The model under review builds one solid part; all positions refer to its coordinate system, in mm. A direction names the side the tool comes from. Give positions to 0.01 mm unless a question says otherwise; leave off trailing zeros. Write each loop counter-clockwise with the first axis right and the second up, starting at its lowest first coordinate (ties: lowest second). Pieces come first, ordered by that corner, then holes.
from build123d import *

# Parameters (mm, degrees)
SKETCH3_R             = 25.4
SKETCH3_R_2           = 20.32
BOSS_EXTRUDE1_DEPTH   = 25.4
BOSS_EXTRUDE3_START   = 7
SKETCH4_R             = 5
BOSS_EXTRUDE3_DEPTH   = 5
BOSS_EXTRUDE3_2_DEPTH = 5
BOSS_EXTRUDE4_START   = -7
SKETCH4_2_R           = 5
BOSS_EXTRUDE4_DEPTH   = 5
BOSS_EXTRUDE4_2_DEPTH = 5
BOSS_EXTRUDE5_DEPTH   = 25.4


with BuildPart() as part:
    # Sketch3 → Boss-Extrude1 (new, symmetric)
    with BuildSketch(Plane(origin=(0, 0, 0), x_dir=(0, 0, -1), z_dir=(1, 0, 0))):
        Circle(SKETCH3_R)
        Circle(SKETCH3_R_2, mode=Mode.SUBTRACT)
    extrude(amount=BOSS_EXTRUDE1_DEPTH, both=True)



with BuildPart() as body_2:
    # Sketch4 → Boss-Extrude3 (new body)
    with BuildSketch(Plane.XY.offset(BOSS_EXTRUDE3_START)):
        with BuildLine():
            Line((-25.4, 25.4), (-9.806723533, 103.556571886))
            ThreePointArc((-9.806723533, 103.556571886), (0, 111.6), (9.806723533, 103.556571886))
            Line((9.806723533, 103.556571886), (25.4, 25.4))
            Line((25.4, 25.4), (-25.4, 25.4))
        make_face()
        with Locations((0, 101.6)):
            Circle(SKETCH4_R, mode=Mode.SUBTRACT)
    extrude(amount=BOSS_EXTRUDE3_DEPTH)


with BuildPart() as body_3:
    # Sketch4 → Boss-Extrude3 2 (new body)
    with BuildSketch(Plane.XY.offset(BOSS_EXTRUDE3_START)):
        with BuildLine():
            Line((-25.4, -25.4), (-9.806723533, -103.556571886))
            ThreePointArc((-9.806723533, -103.556571886), (0, -111.6), (9.806723533, -103.556571886))
            Line((9.806723533, -103.556571886), (25.4, -25.4))
            Line((25.4, -25.4), (-25.4, -25.4))
        make_face()
        with Locations((0, -101.6)):
            Circle(SKETCH4_R, mode=Mode.SUBTRACT)
    extrude(amount=BOSS_EXTRUDE3_2_DEPTH)


with BuildPart() as body_4:
    # Sketch4<2> → Boss-Extrude4 (new body)
    with BuildSketch(Plane.XY.offset(BOSS_EXTRUDE4_START)):
        with BuildLine():
            Line((-25.4, 25.4), (-9.806723533, 103.556571886))
            ThreePointArc((-9.806723533, 103.556571886), (0, 111.6), (9.806723533, 103.556571886))
            Line((9.806723533, 103.556571886), (25.4, 25.4))
            Line((25.4, 25.4), (-25.4, 25.4))
        make_face()
        with Locations((0, 101.6)):
            Circle(SKETCH4_2_R, mode=Mode.SUBTRACT)
    extrude(amount=-BOSS_EXTRUDE4_DEPTH)


with BuildPart() as body_5:
    # Sketch4<2> → Boss-Extrude4 2 (new body)
    with BuildSketch(Plane.XY.offset(BOSS_EXTRUDE4_START)):
        with BuildLine():
            Line((-25.4, -25.4), (-9.806723533, -103.556571886))
            ThreePointArc((-9.806723533, -103.556571886), (0, -111.6), (9.806723533, -103.556571886))
            Line((9.806723533, -103.556571886), (25.4, -25.4))
            Line((25.4, -25.4), (-25.4, -25.4))
        make_face()
        with Locations((0, -101.6)):
            Circle(SKETCH4_2_R, mode=Mode.SUBTRACT)
    extrude(amount=-BOSS_EXTRUDE4_2_DEPTH)


with BuildPart() as part_1:
    add(part.part)

    add(body_2.part)  # Boss-Extrude5 merges body 2

    add(body_3.part)  # Boss-Extrude5 merges body 3

    add(body_4.part)  # Boss-Extrude5 merges body 4

    add(body_5.part)  # Boss-Extrude5 merges body 5
    # Sketch5 → Boss-Extrude5 (add, symmetric)
    with BuildSketch(Plane(origin=(0, 0, 0), x_dir=(0, 0, -1), z_dir=(1, 0, 0))):
        with BuildLine():
            Line((12, -25.4), (7, -25.4))
            Line((7, -25.4), (7, -24.416387939))
            ThreePointArc((7, -24.416387939), (9.554057075, -23.534655158), (12, -22.386603137))
            Line((12, -22.386603137), (12, -25.4))
        make_face()
        with BuildLine():
            Line((-12, -25.4), (-7, -25.4))
            Line((-7, -25.4), (-7, -24.416387939))
            ThreePointArc((-7, -24.416387939), (-9.554057075, -23.534655158), (-12, -22.386603137))
            Line((-12, -22.386603137), (-12, -25.4))
        make_face()
        with BuildLine():
            Line((12, 25.4), (7, 25.4))
            Line((7, 25.4), (7, 24.416387939))
            ThreePointArc((7, 24.416387939), (9.554057075, 23.534655158), (12, 22.386603137))
            Line((12, 22.386603137), (12, 25.4))
        make_face()
        with BuildLine():
            Line((-12, 25.4), (-7, 25.4))
            Line((-7, 25.4), (-7, 24.416387939))
            ThreePointArc((-7, 24.416387939), (-9.554057075, 23.534655158), (-12, 22.386603137))
            Line((-12, 22.386603137), (-12, 25.4))
        make_face()
    extrude(amount=BOSS_EXTRUDE5_DEPTH, both=True)


solid = part_1.part
1) Consider section C-C, the plane z = -2.5. Give the boundary of the cut face in (x, y).
2) Consider section B-B, the plane y = 31. Give the boundary of the cut face in (x, z), then the cut area to 3 significant figures.
3) The part is to be moulded in two halves that separate along Y. For faces 1 (the cylindrical face through (2.688, 105.816, 9.465)), 2 (the cylindrical face through (-0.2, -111.6, 9.5)), 3 (the flat face through (17.5, 65, -9.5)), say which applies: +Y half, -Y half, draft (parallel to the pull), parting line (faces both ways), or undercut.
4) Tool access review of faces 4 (the flat face through (0, -56, -12)), 5 (the cylindrical face through (-0.2, 111.6, -9.5)): name each direction out of +Z, -Z, +X, -X, +Y, -Y from which nothing blocks a thin tool from reaching the whole face with its end or side.
5) Consider section D-D, the plane z = 9. Give the boundary of the cut face in (x, y), then the cut area to 3 significant figures.
6) To check wall thickness, follow probe 1 along Z at (x, y) = (6, -57); probe 2 along Y at (x, z) = (-2.5, 11); probe 3 along Y at (x, z) = (11.5, 0). State the ranges of each line that lie inside material, in increasing order.
7) Insertion check: pin 1 (11.5 mm diameter, centred on x = 0, y = 101.6, fed in from +Z); pin 2 (12 mm diameter, centred on x = -12, y = 70, fed in from -Z); pin 3 (3 mm diameter, centred on y = 67.5, z = -8, fed in from -X). Each pin has a flat end and moves straight along its axis. Give the tip position at first contact, or say it passes through.
8) Consider section A-A, the plane x = 0. State how many separate pieces and enclosed holes the cut face has, then the cut area to 3 significant figures.
Answer block:
1. outline: (-25.4, -25.28) - (25.4, -25.28) - (25.4, -20.17) - (-25.4, -20.17) - close; (-25.4, 20.17) - (25.4, 20.17) - (25.4, 25.28) - (-25.4, 25.28) - close
2. outline: (-24.28, -12) - (24.28, -12) - (24.28, -7) - (-24.28, -7) - close; (-24.28, 7) - (24.28, 7) - (24.28, 12) - (-24.28, 12) - close
2. area: 486 mm2
3. face 1: undercut
3. face 2: -Y half
3. face 3: +Y half
4. face 4: -Z, +X, -X, -Y
4. face 5: +Z, -Z, +Y
5. outline: (-25.4, -25.4) - (-9.81, -103.56) arc R10 ccw to (9.81, -103.56) - (25.4, -25.4) - (25.4, -18.22) - (-25.4, -18.22) - close; (-25.4, 18.22) - (25.4, 18.22) - (25.4, 25.4) - (9.81, 103.56) arc R10 ccw to (-9.81, 103.56) - (-25.4, 25.4) - close; hole circle Ø10 at (0, -101.6); hole circle Ø10 at (0, 101.6)
5. area: 6,310 mm2
6. probe 1: z = -12 to -7, 7 to 12
6. probe 2: y = -111.28 to -105.93, -97.27 to -17.09, 17.09 to 97.27, 105.93 to 111.28
6. probe 3: y = -25.4 to -20.32, 20.32 to 25.4
7. pin 1: stops at z = 12
7. pin 2: stops at z = -12
7. pin 3: stops at x = -17.3
8. separate pieces: 5
8. enclosed holes: 1
8. area: 2,290 mm2
